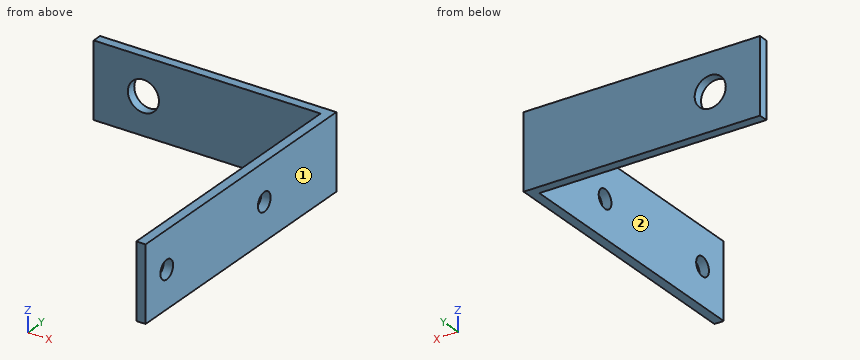
```python
from build123d import *

# Parameters (mm, degrees)
SKETCH1_W           = 36.5
SKETCH1_H           = 12
BOSS_EXTRUDE1_DEPTH = 1.5
SKETCH1_3_W         = 1.5
SKETCH1_3_H         = 12
BOSS_EXTRUDE2_DEPTH = 45
SKETCH2_R           = 1.5
CUT_EXTRUDE1_DEPTH  = 60.203040462
SKETCH3_R           = 2.5
CUT_EXTRUDE2_DEPTH  = 30


with BuildPart() as part:
    # Sketch1 → Boss-Extrude1 (new body)
    with BuildSketch(Plane(origin=(0, 0, 0), x_dir=(1, 0, 0), z_dir=(0, 1, 0))):
        with Locations((-0.75, 0)):
            Rectangle(SKETCH1_W, SKETCH1_H)
    extrude(amount=-BOSS_EXTRUDE1_DEPTH)

    # Sketch1_3 → Boss-Extrude2 (add)
    with BuildSketch(Plane(origin=(0, 0, 0), x_dir=(1, 0, 0), z_dir=(0, 1, 0))):
        with Locations((18.25, 0)):
            Rectangle(SKETCH1_3_W, SKETCH1_3_H)
    extrude(amount=-BOSS_EXTRUDE2_DEPTH)

    # Sketch2 → Cut-Extrude1 (cut, through all)
    with BuildSketch(Plane(origin=(19, 0, 0), x_dir=(0, 0, -1), z_dir=(1, 0, 0))):
        with Locations((0, -40)):
            Circle(SKETCH2_R)
        with Locations((0, -17)):
            Circle(SKETCH2_R)
    extrude(amount=-CUT_EXTRUDE1_DEPTH, mode=Mode.SUBTRACT)

    # Sketch3 → Cut-Extrude2 (cut)
    with BuildSketch(Plane(origin=(0, 0, 0), x_dir=(1, 0, 0), z_dir=(0, 1, 0))):
        with Locations(Location((-11, 0, 0), (0, 0, 270))):
            Circle(SKETCH3_R)
    extrude(amount=-CUT_EXTRUDE2_DEPTH, mode=Mode.SUBTRACT)


solid = part.part
```
Source: CAD feature listing. Evaluate the final solid. Frame: model axes, mm. Face numbers are marked on the shaded views. A direction names the side the tool comes from. Round coordinates to 2 decimals unless told otherwise and drop trailing zeros. Write each loop counter-clockwise with the first axis right and the second up, starting at its lowest first coordinate (ties: lowest second). Pieces come first, ordered by that corner, then holes. Notation, with made-up numbers: M -12,-7 L 11,-7 A21 cw 11,11 Z; hole C 15.25,-27 d9. An arc over 180 degrees is marked long. Answer as a JSON object with one key per item and string values. Group by question number.
(1) Section query C-C on y = -40. Output: boundary loops of the cut face in (x, z), then the cut area to 3 significant figures.
(2) Ray query, line 1 (Y direction, x = 18.2, z = 0); line 2 (X direction, y = -0.4, z = 0); line 3 (Y direction, x = 9.5, z = 2.5). Return the intervals inside material, ascending. Write a range as [from, to].
(3) Section query A-A on x = -11. Output: boundary loops of the cut face in (y, z), then the cut area to 3 significant figures.
(4) Reachability of the marked faces 1 and 2 from +Z, -Z, +X, -X, +Y, -Y: full face, straight path, thin tool, end or side. Return the list, or none.
(5) Section query D-D on y = -22. Output: boundary loops of the cut face in (x, z), then the cut area to 3 significant figures.
(6) First-contact query: pin 1 (3 mm diameter, centred on y = -24, z = 0.5, fed in from -X); pin 2 (4.5 mm diameter, centred on x = -11, z = 0, fed in from -Y); pin 3 (3 mm diameter, centred on x = -7.5, z = 3, fed in from -Y). Flat tips, straight axial feed; report the tip coordinate or a pass-through.
(7) Section query B-B on z = 0. Output: boundary loops of the cut face in (x, y).
Computed values:
{
 "1": {"outline": "M 17.5,-6 L 19,-6 L 19,-1.5 L 17.5,-1.5 Z; M 17.5,1.5 L 19,1.5 L 19,6 L 17.5,6 Z", "area": "13.5 mm^2"},
 "2": {"line 1": "[-45, -41.5], [-38.5, -18.5], [-15.5, 0]", "line 2": "[-19, -13.5], [-8.5, 19]", "line 3": "[-1.5, 0]"},
 "3": {"outline": "M -1.5,-6 L 0,-6 L 0,-2.5 L -1.5,-2.5 Z; M -1.5,2.5 L 0,2.5 L 0,6 L -1.5,6 Z", "area": "10.5 mm^2"},
 "4": {"face 1": "+Z, -Z, +X, +Y, -Y", "face 2": "+Z, -Z, -X, -Y"},
 "5": {"outline": "M 17.5,-6 L 19,-6 L 19,6 L 17.5,6 Z", "area": "18.0 mm^2"},
 "6": {"pin 1": "x = 17.5", "pin 2": "through", "pin 3": "y = -1.5"},
 "7": {"outline": "M -19,-1.5 L -13.5,-1.5 L -13.5,0 L -19,0 Z; M -8.5,-1.5 L 17.5,-1.5 L 17.5,-15.5 L 19,-15.5 L 19,0 L -8.5,0 Z; M 17.5,-45 L 19,-45 L 19,-41.5 L 17.5,-41.5 Z; M 17.5,-38.5 L 19,-38.5 L 19,-18.5 L 17.5,-18.5 Z"}
}
